from build123d import *

# Parameters (mm, degrees)
F1_DEPTH = 3
F2_W     = 10
F2_H     = 5.5
F3_DEPTH = 25
F4_W     = 3.02
F4_H     = 2.9
F5_DEPTH = 25


with BuildPart() as f1:
    # F0 (on Right) → F1 (new body)
    with BuildSketch(Plane.YZ):
        Polygon((80, 30), (0, 30), (-80, 30), (-80, -30), (0, -30), (80, -30), align=None)
    extrude(amount=F1_DEPTH)

    # F2 (on face) → F3 (cut)
    with BuildSketch(Plane.YZ.offset(3)):
        with Locations((-55, -4.25)):
            Rectangle(F2_W, F2_H)
        with Locations((-55, 4.25)):
            Rectangle(F2_W, F2_H)
        with Locations((55, 4.25)):
            Rectangle(F2_W, F2_H)
        with Locations((55, -4.25)):
            Rectangle(F2_W, F2_H)
    extrude(amount=-F3_DEPTH, mode=Mode.SUBTRACT)

    # F4 (on face) → F5 (cut)
    with BuildSketch(Plane.YZ.offset(3)):
        with Locations((-4.346554, 24.356653)):
            Rectangle(F4_W, F4_H)
        with Locations((4.346554, 24.356653)):
            Rectangle(F4_W, F4_H)
    extrude(amount=-F5_DEPTH, mode=Mode.SUBTRACT)


solid = f1.part
Read the model definition and answer for the solid it produces. Units are mm, in the model's axes. Give positions to 0.01 mm unless a question says otherwise; leave off trailing zeros. Write each loop counter-clockwise with the first axis right and the second up, starting at its lowest first coordinate (ties: lowest second). Pieces come first, ordered by that corner, then holes. Notation, with made-up numbers: (46, 84.25) -> (53, 84.25) arc R17 ccw to (53, 117.25) -> close; hole circle Ø7 at (-40, -31). An arc over 180 degrees is marked (long way). Answer as a JSON object with one key per item and string values. Group by question number.
1) Find section B-B (z = 4.5). Write down the section's boundary in (x, y).
2) This flat-tipped pin is pushed along its axis until it touches: P1, Ø1.5, axis at y = 53.5, z = -1.5, coming from the -X side. Where does it stop, or does it pass through?
3) Find section A-A (y = 52.5). Write down the section's boundary in (x, z), and give its area (3 significant figures).
4) The mould has two halves that part along Z. Classify faces 1 (the flat face through (2, -60, -4)), 2 (the flat face through (1, -1, -30)), 3 (the flat face through (1, -80, 0)), 4 (the flat face through (1, 1, 30)): +Z half, -Z half, draft (parallel to the pull), parting line (faces both ways), or undercut.
5) Find section C-C (x = 2.55). Write down the section's boundary in (y, z), and give its area (3 significant figures).
6) Consider L1, parallel to Z at x = 2.5, y = -53.5; L2, parallel to Y at x = 1.75, z = -2.5; L3, parallel to Y at x = 2.75, z = 25. Determine where each line is inside the solid, lowest interval first. Write a range as from..to.
Values follow:
{
 "1": {"outline": "(0, -80) -> (3, -80) -> (3, -60) -> (0, -60) -> close; (0, -50) -> (3, -50) -> (3, 50) -> (0, 50) -> close; (0, 60) -> (3, 60) -> (3, 80) -> (0, 80) -> close"},
 "2": {"P1": "stops at x = 0"},
 "3": {"outline": "(0, -30) -> (3, -30) -> (3, -7) -> (0, -7) -> close; (0, -1.5) -> (3, -1.5) -> (3, 1.5) -> (0, 1.5) -> close; (0, 7) -> (3, 7) -> (3, 30) -> (0, 30) -> close", "area": "147 mm2"},
 "4": {"face 1": "undercut", "face 2": "-Z half", "face 3": "draft", "face 4": "+Z half"},
 "5": {"outline": "(-80, -30) -> (80, -30) -> (80, 30) -> (-80, 30) -> close; hole (-60, -7) -> (-50, -7) -> (-50, -1.5) -> (-60, -1.5) -> close; hole (-60, 1.5) -> (-50, 1.5) -> (-50, 7) -> (-60, 7) -> close; hole (-5.86, 22.91) -> (-2.84, 22.91) -> (-2.84, 25.81) -> (-5.86, 25.81) -> close; hole (2.84, 22.91) -> (5.86, 22.91) -> (5.86, 25.81) -> (2.84, 25.81) -> close; hole (50, -7) -> (60, -7) -> (60, -1.5) -> (50, -1.5) -> close; hole (50, 1.5) -> (60, 1.5) -> (60, 7) -> (50, 7) -> close", "area": "9,360 mm2"},
 "6": {"L1": "z = -30..-7, -1.5..1.5, 7..30", "L2": "y = -80..-60, -50..50, 60..80", "L3": "y = -80..-5.86, -2.84..2.84, 5.86..80"}
}
